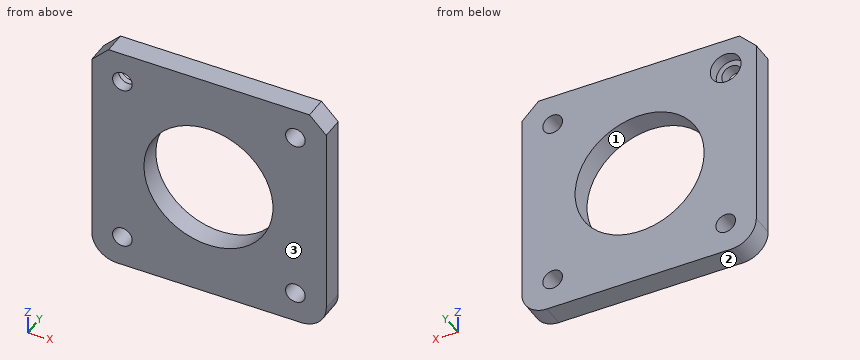
Autodesk Inventor part; units mm, degrees
ref_plane "YZ Plane" through (0, 0, 0) normal (1, 0, 0) x (0, 1, 0)
ref_plane "XZ Plane" through (0, 0, 0) normal (0, 1, 0) x (-1, 0, 0)
ref_plane "XY Plane" through (0, 0, 0) normal (0, 0, 1) x (1, 0, 0)
sketch "Sketch1" plane through (0, 0, 0) normal (0, 1, 0) x (-1, 0, 0)
  circle A0 centre (0, 0) radius 11.56
  line L0 (20.9, -21.04) -> (-21.11, -21.04)
  line L1 (20.9, 20.96) -> (-21.11, 20.96)
  line L2 (20.9, 20.96) -> (20.9, -21.04)
  line L3 (-21.11, 20.96) -> (-21.11, -21.04)
  dimension "d1" = 23.12
  dimension "d2" = 21.04
  dimension "d3" = 20.9
  dimension "d4" = 20.96
  dimension "d5" = 21.11
extrude "Extrusion1" add sketch "Sketch1" along normal blind 4.02
sketch "Sketch2" plane through (0, 4.02, 0) normal (0, 1, 0) x (1, 0, 0)
  point P0 (0, 0)
  point P1 (15.58, -15.48)
  point P2 (15.58, 15.52)
  point P3 (-15.42, 15.52)
  point P4 (-15.42, -15.48)
  dimension "d8" = 15.52
  dimension "d9" = 15.48
  dimension "d10" = 15.42
  dimension "d11" = 15.58
hole "Hole1" at (15.58, 4.02, 15.48) at (15.58, 4.02, -15.52) at (-15.42, 4.02, -15.52) direction (0, -1, 0) diameter 3.52 end through all
hole "Hole2" at (-15.42, 4.02, 15.48) direction (0, -1, 0) diameter 3.52 end through all counterbore diameter 5.52 counterbore depth 2
fillet "Fillet1" radius 4.5 2 edges at (-20.9, 2.01, -21.04) (21.11, 2.01, -21.04)
chamfer "Chamfer1" distance 3 angle 45 2 edges at (-20.9, 2.01, 20.96) (21.11, 2.01, 20.96)
properties part number "Extruder Housing"
Geometry check sheet. Reference: the model listing, model coordinates, mm. Face numbers are marked on the shaded views. Round coordinates to 2 decimals unless told otherwise and drop trailing zeros. Order: outer loops, then holes, each group sorted by start corner. A loop starts at its lowest first (then second) coordinate and runs counter-clockwise, first axis right, second up. Notation, with made-up numbers: M 62,-14 L 114,-14 A27 cw 114,21 Z; hole C 73.5,-23 d6. An arc over 180 degrees is marked long. Answer as CSV lines item,"result".
1) Sectioned sample at B-B on x = 0. Record the cut outline in (y, z), and give its area (3 significant figures).
Entries:
outline,"M 0,-21.04 L 4.02,-21.04 L 4.02,-11.56 L 0,-11.56 Z; M 0,11.56 L 4.02,11.56 L 4.02,20.96 L 0,20.96 Z"
area,"75.9 mm2"
2) Thickness scan on probe 1 along X at (y, z) = (1.15, 15.48); probe 2 along Z at (x, y) = (-15.42, 1.05); probe 3 along X at (y, z) = (2.1, 15.48). Record the ranges inside material, lowest first. Write a range as [from, to].
Entries:
probe 1,"[-20.9, -17.18], [-13.66, 13.82], [17.34, 21.11]"
probe 2,"[-21.04, -17.28], [-13.76, 13.72], [17.24, 20.96]"
probe 3,"[-20.9, -18.18], [-12.66, 13.82], [17.34, 21.11]"
3) Sectioned sample at A-A on z = 15.48. Record the cut outline in (x, y).
Entries:
outline,"M -20.9,0 L -17.18,0 L -17.18,2.02 L -18.18,2.02 L -18.18,4.02 L -20.9,4.02 Z; M -13.66,0 L 13.82,0 L 13.82,4.02 L -12.66,4.02 L -12.66,2.02 L -13.66,2.02 Z; M 17.34,0 L 21.11,0 L 21.11,4.02 L 17.34,4.02 Z"
4) Sectioned sample at D-D on x = -15.42. Record the cut outline in (y, z), and give its area (3 significant figures).
Entries:
outline,"M 0,-21.04 L 4.02,-21.04 L 4.02,-17.28 L 0,-17.28 Z; M 0,-13.76 L 4.02,-13.76 L 4.02,12.72 L 2.02,12.72 L 2.02,13.72 L 0,13.72 Z; M 0,17.24 L 2.02,17.24 L 2.02,18.24 L 4.02,18.24 L 4.02,20.96 L 0,20.96 Z"
area,"137 mm2"
5) Sectioned sample at C-C on y = 1.2. Record the cut outline in (x, z), and give its area (3 significant figures).
Entries:
outline,"M -20.9,-16.54 A4.5 ccw -16.4,-21.04 L 16.61,-21.04 A4.5 ccw 21.11,-16.54 L 21.11,17.96 L 18.11,20.96 L -17.9,20.96 L -20.9,17.96 Z; hole C -15.42,-15.52 d3.52; hole C -15.42,15.48 d3.52; hole C 0,0 d23.12; hole C 15.58,-15.52 d3.52; hole C 15.58,15.48 d3.52"
area,"1,290 mm2"
6) Mould release check, pull along Z, two halves, no side actions. Record for the marked faces 1, 2 and 3: +Z half, -Z half, draft (parallel to the pull), parting line (faces both ways), or undercut.
Entries:
face 1,"undercut"
face 2,"-Z half"
face 3,"draft"
7) Gauge pin test, flat end, axial feed: pin 1 Ø4.5 at (x, z) = (-15.42, 15.48) entering from +Y. Record the tip position at first contact, or that the pin passes through.
Entries:
pin 1,"y = 2.02"
